Source: CAD feature listing. Evaluate the final solid. Frame: model axes, mm. A direction names the side the tool comes from. Give positions to 0.01 mm unless a question says otherwise; leave off trailing zeros. Loops run counter-clockwise (first coordinate to the right, second up) from the corner with the lowest first, then second, coordinate; pieces in that order, holes last. Notation, with made-up numbers: (49.5, 38.5) - (70.5, 38.5) arc R35 cw to (70.5, 75.5) - close; hole circle Ø11 at (81.5, 23). An arc over 180 degrees is marked (long way). Put each result on its own line as item: value.
```python
from build123d import *

# Parameters (mm, degrees)
BOSS_EXTRUDE1_DEPTH = 50
SKETCH2_R           = 10
CUT_EXTRUDE1_DEPTH  = 50
SKETCH3_R           = 30
BOSS_EXTRUDE2_DEPTH = 30
SKETCH4_R           = 20
CUT_EXTRUDE2_DEPTH  = 20
SKETCH5_R           = 10
CUT_EXTRUDE3_DEPTH  = 20
SKETCH6_W           = 40
SKETCH6_H           = 10
CUT_EXTRUDE4_DEPTH  = 20
SKETCH7_W           = 40
SKETCH7_H           = 10
CUT_EXTRUDE5_DEPTH  = 20
SKETCH8_W           = 40
SKETCH8_H           = 10
CUT_EXTRUDE6_DEPTH  = 20
SKETCH9_W           = 40
SKETCH9_H           = 10
CUT_EXTRUDE7_DEPTH  = 20
SKETCH10_R          = 10
CUT_EXTRUDE8_DEPTH  = 60
SKETCH11_R          = 10
CUT_EXTRUDE9_DEPTH  = 20


with BuildPart() as part:
    # Sketch1 → Boss-Extrude1 (new body)
    with BuildSketch(Plane.XY):
        with BuildLine():
            Line((0, 50), (60, 50))
            ThreePointArc((60, 50), (110, 0), (60, -50))
            Line((60, -50), (0, -50))
            ThreePointArc((0, -50), (-50, 0), (0, 50))
        make_face()
    extrude(amount=BOSS_EXTRUDE1_DEPTH)

    # Sketch2 → Cut-Extrude1 (cut)
    with BuildSketch(Plane.XY.offset(50)):
        with Locations((30, 0)):
            Circle(SKETCH2_R)
    extrude(amount=-CUT_EXTRUDE1_DEPTH, mode=Mode.SUBTRACT)

    # Sketch3 → Boss-Extrude2 (add)
    with BuildSketch(Plane.XY.offset(50)):
        with Locations((30, 0)):
            Circle(SKETCH3_R)
    extrude(amount=BOSS_EXTRUDE2_DEPTH)

    # Sketch4 → Cut-Extrude2 (cut)
    with BuildSketch(Plane.XY.offset(80)):
        with Locations((30, 0)):
            Circle(SKETCH4_R)
    extrude(amount=-CUT_EXTRUDE2_DEPTH, mode=Mode.SUBTRACT)

    # Sketch5 → Cut-Extrude3 (cut)
    with BuildSketch(Plane(origin=(0, 0, 50), x_dir=(-1, 0, 0), z_dir=(0, 0, -1))):
        with Locations((-30, 0)):
            Circle(SKETCH5_R)
    extrude(amount=-CUT_EXTRUDE3_DEPTH, mode=Mode.SUBTRACT)

    # Sketch6 → Cut-Extrude4 (cut)
    with BuildSketch(Plane.XY.offset(50)):
        with Locations((30, 45)):
            Rectangle(SKETCH6_W, SKETCH6_H)
    extrude(amount=-CUT_EXTRUDE4_DEPTH, mode=Mode.SUBTRACT)

    # Sketch7 → Cut-Extrude5 (cut)
    with BuildSketch(Plane(origin=(0, 0, 0), x_dir=(-1, 0, 0), z_dir=(0, 0, -1))):
        with Locations((-30, 45)):
            Rectangle(SKETCH7_W, SKETCH7_H)
    extrude(amount=-CUT_EXTRUDE5_DEPTH, mode=Mode.SUBTRACT)

    # Sketch8 → Cut-Extrude6 (cut)
    with BuildSketch(Plane.XY.offset(50)):
        with Locations((30, -45)):
            Rectangle(SKETCH8_W, SKETCH8_H)
    extrude(amount=-CUT_EXTRUDE6_DEPTH, mode=Mode.SUBTRACT)

    # Sketch9 → Cut-Extrude7 (cut)
    with BuildSketch(Plane(origin=(0, 0, 0), x_dir=(-1, 0, 0), z_dir=(0, 0, -1))):
        with Locations((-30, -45)):
            Rectangle(SKETCH9_W, SKETCH9_H)
    extrude(amount=-CUT_EXTRUDE7_DEPTH, mode=Mode.SUBTRACT)

    # Sketch10 → Cut-Extrude8 (cut)
    with BuildSketch(Plane.XY.offset(50)):
        with Locations((-30, 0)):
            Circle(SKETCH10_R)
        with Locations((90, 0)):
            Circle(SKETCH10_R)
    extrude(amount=-CUT_EXTRUDE8_DEPTH, mode=Mode.SUBTRACT)

    # Sketch11 → Cut-Extrude9 (cut)
    with BuildSketch(Plane.XY.offset(50)):
        with BuildLine():
            ThreePointArc((-30, -20), (-10, 0), (-30, 20))
            Line((-30, 20), (-45.82575695, 20))
            ThreePointArc((-45.82575695, 20), (-50, 0), (-45.82575695, -20))
            Line((-45.82575695, -20), (-30, -20))
        make_face()
        with Locations((-30, 0)):
            Circle(SKETCH11_R, mode=Mode.SUBTRACT)
        with BuildLine():
            Line((105.82575695, 20), (90, 20))
            ThreePointArc((90, 20), (70, 0), (90, -20))
            Line((90, -20), (105.82575695, -20))
            ThreePointArc((105.82575695, -20), (110, 0), (105.82575695, 20))
        make_face()
        with Locations((90, 0)):
            Circle(SKETCH11_R, mode=Mode.SUBTRACT)
    extrude(amount=-CUT_EXTRUDE9_DEPTH, mode=Mode.SUBTRACT)


solid = part.part
```
1) Access query for faces 1 (the flat face through (50, 45, 10)), 2 (the flat face through (30, 45, 30)), 3 (the flat face through (50, -45, 10)). Directions: +Z, -Z, +X, -X, +Y, -Y. A direction counts if a zero-diameter tool reaches every point of the face in a straight line with its end or side. Return the directions, or none.
Check result:
face 1: -Z, +Y
face 2: +Z, +Y
face 3: -Z, -Y
2) Section query C-C, the plane z = 33. Output: boundary loops of the cut face in (x, y).
Check result:
outline: (-45.83, -20) arc R50 ccw to (0, -50) - (10, -50) - (10, -40) - (50, -40) - (50, -50) - (60, -50) arc R50 ccw to (105.83, -20) - (90, -20) arc R20 cw to (90, 20) - (105.83, 20) arc R50 ccw to (60, 50) - (50, 50) - (50, 40) - (10, 40) - (10, 50) - (0, 50) arc R50 ccw to (-45.83, 20) - (-30, 20) arc R20 cw to (-30, -20) - close; hole circle Ø20 at (30, 0)
3) Section query B-B, the plane y = -8. Output: boundary loops of the cut face in (x, z), plus the area to 3 significant figures.
Check result:
outline: (-49.36, 0) - (-36, 0) - (-36, 30) - (-49.36, 30) - close; (-24, 0) - (24, 0) - (24, 60) - (11.67, 60) - (11.67, 80) - (1.09, 80) - (1.09, 50) - (-11.67, 50) - (-11.67, 30) - (-24, 30) - close; (36, 0) - (84, 0) - (84, 30) - (71.67, 30) - (71.67, 50) - (58.91, 50) - (58.91, 80) - (48.33, 80) - (48.33, 60) - (36, 60) - close; (96, 0) - (109.36, 0) - (109.36, 30) - (96, 30) - close
area: 5,990 mm²
4) Section query D-D, the plane x = 93. Output: boundary loops of the cut face in (y, z), plus the area to 3 significant figures.
Check result:
outline: (-37.56, 0) - (-9.54, 0) - (-9.54, 30) - (-20, 30) - (-20, 50) - (-37.56, 50) - close; (9.54, 0) - (37.56, 0) - (37.56, 50) - (20, 50) - (20, 30) - (9.54, 30) - close
area: 2,380 mm²
5) Pin query (flat end, axial travel): P1, Ø1, axis at x = -27.5, y = 18.5, coming from the +Z side; P2, Ø8, axis at y = 47, z = 9, coming from the -X side; P3, Ø5, axis at x = -23.5, y = 32.5, coming from the -Z side; P4, Ø8, axis at y = 44, z = 5.5, coming from the +X side. Return the tip coordinate at first contact, or that it passes through.
Check result:
P1: z = 30
P2: x = -25.51
P3: z = 0
P4: x = 90
6) Mould query, pull axis X, two halves, no side actions, for faces 4 (the flat face through (30, -40, 40)), 5 (the cylindrical face through (0.03, 1.32, 64.79)), 6 (the flat face through (-38, 20, 40)). Classes: pulls with the +X half, pulls with the -X half, needs draft (parallel to the pull), parting line crosses it, or undercut.
Check result:
face 4: undercut
face 5: parting line crosses it
face 6: needs draft
7) Material intervals for line 1 along Y through (x, z) = (30, 55.25); line 2 along Y through (x, z) = (30, 14.5); line 3 along X through (y, z) = (7.5, 44), sorted ascending. Write a range as [from, to].
Check result:
line 1: [-30, -10], [10, 30]
line 2: [-40, -10], [10, 40]
line 3: [-11.46, 23.39], [36.61, 71.46]
8) Section query A-A, the plane x = 30. Output: boundary loops of the cut face in (y, z), plus the area to 3 significant figures.
Check result:
outline: (-50, 20) - (-40, 20) - (-40, 0) - (-10, 0) - (-10, 60) - (-20, 60) - (-20, 80) - (-30, 80) - (-30, 50) - (-40, 50) - (-40, 30) - (-50, 30) - close; (10, 0) - (40, 0) - (40, 20) - (50, 20) - (50, 30) - (40, 30) - (40, 50) - (30, 50) - (30, 80) - (20, 80) - (20, 60) - (10, 60) - close
area: 4,000 mm²
